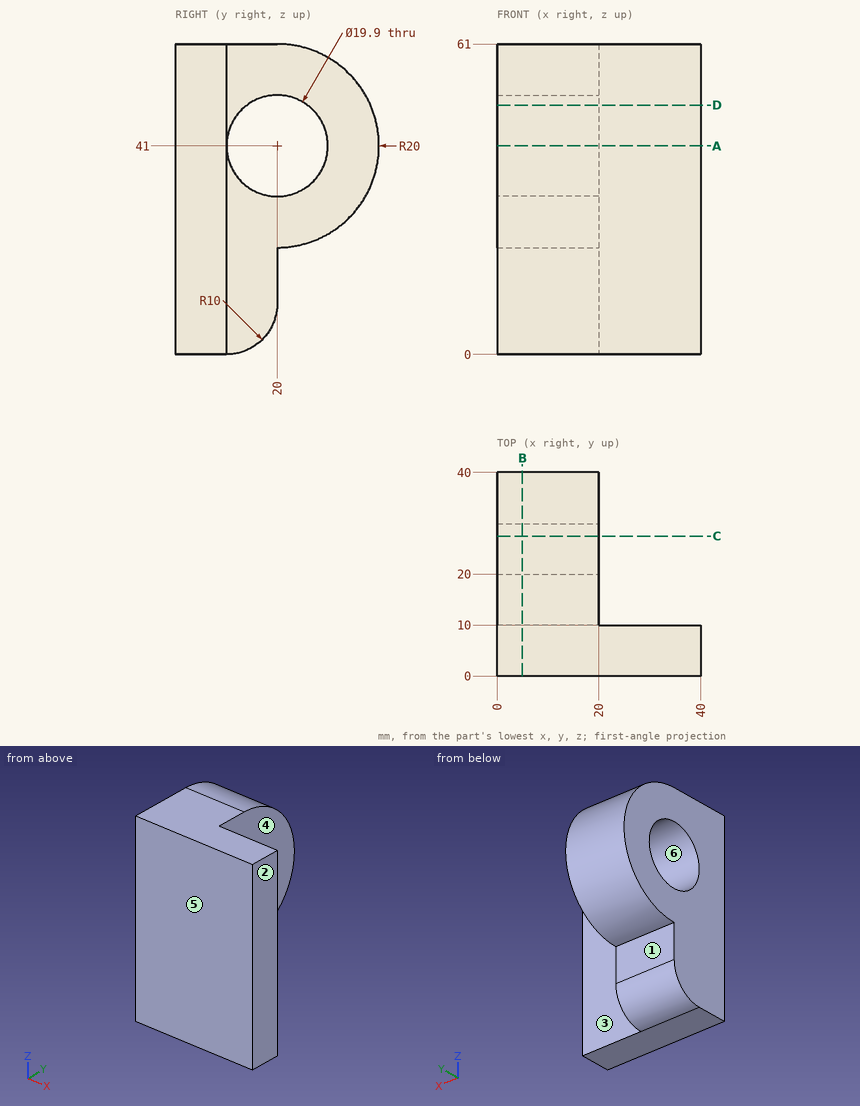
Part print with two shaded views. Sizes in mm from the minimum x, y, z corner. A direction names the side the tool comes from. Coordinates: 2 decimals unless noted, no trailing zeros. Write each loop counter-clockwise with the first axis right and the second up, starting at its lowest first coordinate (ties: lowest second). Pieces come first, ordered by that corner, then holes. Notation, with made-up numbers: M 69.25,-37.5 L 107.25,-37.5 A11 cw 107.25,-19.5 Z; hole C 37,-29 d1. An arc over 180 degrees is marked long. Return JSON: item names as keys, results as strings.
Item 1: Two-plate mould, pull along Y, no slides. Class the marked faces 4, 5 and 6: +Y half, -Y half, draft (parallel to the pull), parting line (faces both ways), or undercut.
Findings below:
{"face 4": "draft", "face 5": "-Y half", "face 6": "undercut"}
Item 2: Drop flat-ended pins along their axis: pin 1 Ø1 at (y, z) = (29, 52.5) entering from -X; pin 2 Ø12 at (x, y) = (32, 21.5) entering from +Z; pin 3 Ø5.5 at (x, z) = (6.5, 13.5) entering from +Y; pin 4 Ø10 at (x, z) = (33, 34) entering from +Y. Give the stop position or say it passes through.
Findings below:
{"pin 1": "stops at x = 0", "pin 2": "passes through", "pin 3": "stops at y = 20", "pin 4": "stops at y = 10"}
Item 3: Slice it at B-B, the plane x = 5. Write the cut outline in (y, z), and give its area (3 significant figures).
Findings below:
{"outline": "M 0,0 L 10,0 A10 ccw 20,10 L 20,21 A20 ccw 20,61 L 0,61 Z; hole C 20,41 d19.9", "area": "1,520 mm2"}
Item 4: Probe line 1 (Y direction, x = 11.25, z = 41); line 2 (X direction, y = 12, z = 25); line 3 (Y direction, x = 34, z = 52). List the from-to ranges inside material, lowest first. Write a range as from..to.
Findings below:
{"line 1": "y = 0..10.05, 29.95..40", "line 2": "x = 0..20", "line 3": "y = 0..10"}
Item 5: Slice it at D-D, the plane z = 49. Write the cut outline in (x, y).
Findings below:
{"outline": "M 0,0 L 40,0 L 40,10 L 20,10 L 20,14.08 L 0,14.08 Z; M 0,25.92 L 20,25.92 L 20,38.33 L 0,38.33 Z"}
Item 6: Slice it at C-C, the plane y = 27.5. Write the cut outline in (x, z), and give its area (3 significant figures).
Findings below:
{"outline": "M 0,22.46 L 20,22.46 L 20,34.46 L 0,34.46 Z; M 0,47.54 L 20,47.54 L 20,59.54 L 0,59.54 Z", "area": "480 mm2"}
Item 7: Slice it at A-A, the plane z = 41. Write the cut outline in (x, y).
Findings below:
{"outline": "M 0,0 L 40,0 L 40,10 L 20,10 L 20,10.05 L 0,10.05 Z; M 0,29.95 L 20,29.95 L 20,40 L 0,40 Z"}
Item 8: Which spindle directions (+Z, -Z, +X, -X, +Y, -Y) get a long thin tool onto all of the face, cutting with end or side? Do the marked faces 1, 2 and 3. Say none if no direction does.
Findings below:
{"face 1": "-Z, +X, -X, +Y", "face 2": "+Z, -Z, +X, +Y, -Y", "face 3": "+Z, -Z, +X, +Y"}
